```python
from build123d import *

# Parameters (mm, degrees)
SKETCH1_R                = 6
BOSS_EXTRUDE1_DEPTH      = 30
BOSS_EXTRUDE2_DEPTH      = 23
BOSS_EXTRUDE2_DEPTH_BACK = 4
SKETCH2_R                = 14
SKETCH2_R_2              = 11


with BuildPart() as part:
    # Sketch1 → Boss-Extrude1 (new body)
    with BuildSketch(Plane(origin=(0, 0, 0), x_dir=(1, 0, 0), z_dir=(0, 1, 0))):
        with BuildLine():
            ThreePointArc((7.652602621, 5.263157895), (0, 19), (-7.652602621, 5.263157895))
            ThreePointArc((-7.652602621, 5.263157895), (-6.155494421, 0), (-7.652602621, -5.263157895))
            ThreePointArc((-7.652602621, -5.263157895), (0, -19), (7.652602621, -5.263157895))
            ThreePointArc((7.652602621, -5.263157895), (6.155494421, 0), (7.652602621, 5.263157895))
        make_face()
        with Locations(Location((0, 10, 0), (0, 0, 270))):
            Circle(SKETCH1_R, mode=Mode.SUBTRACT)
        with Locations(Location((0, -10, 0), (0, 0, 270))):
            Circle(SKETCH1_R, mode=Mode.SUBTRACT)
    extrude(amount=BOSS_EXTRUDE1_DEPTH)

    # Sketch2 → Boss-Extrude2 (add, two sides: drawn at the far end of the back side and taken through both)
    with BuildSketch(Plane(origin=(10, 0, 0), x_dir=(0, 0, -1), z_dir=(1, 0, 0)).offset(-BOSS_EXTRUDE2_DEPTH_BACK)):
        with Locations(Location((0, 15, 0), (0, 0, 112.082413194))):
            Circle(SKETCH2_R)
        with Locations(Location((0, 15, 0), (0, 0, 118.585451093))):
            Circle(SKETCH2_R_2, mode=Mode.SUBTRACT)
    extrude(amount=BOSS_EXTRUDE2_DEPTH + BOSS_EXTRUDE2_DEPTH_BACK)


solid = part.part
```
Could you check a few things on this model? Use its own coordinates, in mm. A direction names the side the tool comes from. Round coordinates to 2 decimals unless told otherwise and drop trailing zeros. Loops run counter-clockwise (first coordinate to the right, second up) from the corner with the lowest first, then second, coordinate; pieces in that order, holes last.
Q1. For P1, Ø5, axis at x = -3.5, z = 5.5, coming from the +Y side; P2, Ø17.5, axis at y = 15, z = 0, coming from the -X side; P3, Ø12, axis at x = 17.5, y = 12.5, coming from the -Z side; P4, Ø3, axis at x = -4, y = 13, coming from the -Z side, each with a flat end and sliding along its axis, tell me the tip position at first contact or that it passes through.
Q2. I want a section at C-C (y = 22.5). Write out the boundary of the cut face in (x, z), and give its area (3 significant figures).
Q3. On a 3-axis mill with a long thin cutter (end or side, diameter ignored), from which of +Z, -Z, +X, -X, +Y, -Y can I reach the whole of each face in a straight line? I mean faces 3 (the cylindrical face through (1.802, 14.79, -4.277)), 4 (the cylindrical face through (6.156, 14.846, 0.078)), 5 (the cylindrical face through (6.156, 0.774, 0.078)), 6 (the cylindrical face through (6.156, 29.198, 0.078)), 7 (the flat face through (0, 0, 0)). Say none if no direction works.
Q4. Thinking about a two-plate mould opening in Z: for faces 1 (the flat face through (0, 30, 0)), 2 (the cylindrical face through (19.39, 5.119, -4.833)), which applies, pulls with the +Z half, pulls with the -Z half, needs draft (parallel to the pull), parting line crosses it, or undercut?
Q5. I want a section at D-D (z = 0). Write out the boundary of the cut face in (x, y), and give its area (3 significant figures).
Q6. Please list where these lines run through material, in increasing order: L1, parallel to Y at x = 17.5, z = -0.5; L2, parallel to X at y = 8.75, z = -10; L3, parallel to Z at x = 22, y = 15.
Q7. I want a section at A-A (x = 0). Write out the boundary of the cut face in (y, z), and give its area (3 significant figures).
Q8. I want a section at B-B (z = 10). Write out the boundary of the cut face in (x, y).
Answer below:
1. P1: stops at y = 30
1. P2: stops at x = -8.91
1. P3: stops at z = -14
1. P4: stops at z = -18.65
2. outline: (-7.65, -5.26) arc R9 ccw (long way) to (8.81, -11.82) - (33, -11.82) - (33, -8.05) - (8.79, -8.05) arc R9 ccw to (7.65, -5.26) arc R10 cw to (7.65, 5.26) arc R9 ccw to (8.79, 8.05) - (33, 8.05) - (33, 11.82) - (8.81, 11.82) arc R9 ccw (long way) to (-7.65, 5.26) arc R10 cw to start; hole circle Ø12 at (0, -10); hole circle Ø12 at (0, 10)
2. area: 512 mm2
3. face 3: +Y, -Y
3. face 4: +X
3. face 5: +X, -Y
3. face 6: +X, +Y
3. face 7: +Z, -Z, +X, -X, -Y
4. face 1: needs draft
4. face 2: undercut
5. outline: (-6.16, 0) - (6.16, 0) - (6.16, 1) - (33, 1) - (33, 4) - (6.16, 4) - (6.16, 26) - (33, 26) - (33, 29) - (6.16, 29) - (6.16, 30) - (-6.16, 30) - close
5. area: 530 mm2
6. L1: y = 1.01 to 4.01, 25.99 to 28.99
6. L2: x = -9 to -6, 6 to 33
6. L3: z = -14 to -11, 11 to 14
7. outline: (0, -19) - (30, -19) - (30, -16) - (0, -16) - close; (0, -4) - (30, -4) - (30, 4) - (0, 4) - close; (0, 16) - (30, 16) - (30, 19) - (0, 19) - close
7. area: 420 mm2
8. outline: (-9, 0) - (-6, 0) - (-6, 30) - (-9, 30) - close; (6, 0) - (9, 0) - (9, 5.2) - (33, 5.2) - (33, 10.42) - (9, 10.42) - (9, 19.58) - (33, 19.58) - (33, 24.8) - (9, 24.8) - (9, 30) - (6, 30) - close
